Can you work these out from the drawing? Everything is in mm from the part's minimum corner. A direction names the side the tool comes from. Coordinates: 2 decimals unless noted, no trailing zeros. Loops run counter-clockwise (first coordinate to the right, second up) from the corner with the lowest first, then second, coordinate; pieces in that order, holes last. Notation, with made-up numbers: (-4.5, 70) - (42.5, 70) arc R16 cw to (42.5, 97) - close; hole circle Ø1 at (34, -26). An arc over 180 degrees is marked (long way). One line per question, with ' | ' between items. Start each with the question number.
1. I want a section at A-A, the plane x = 82. Write out the boundary of the cut face in (y, z), then the cut area to 3 significant figures.
2. I'm going to push a flat-ended pin straight in: P1, Ø5, axis at x = 55.5, y = 41.5, coming from the +Z side. Where does the tip first touch, or does it pass through?
3. Which directions (+Z, -Z, +X, -X, +Y, -Y) give clear straight access to the entire face, cutting with the end or side of a thin tool? Please do the marked faces 1 and 2.
4. We'd pull the mould along Y, two halves only. Please class the marked faces 3, 4 and 5: pulls with the +Y half, pulls with the -Y half, needs draft (parallel to the pull), parting line crosses it, or undercut.
5. I want a section at C-C, the plane z = 10.5. Write out the boundary of the cut face in (x, y).
6. Please list where these lines run through material, in increasing order: L1, parallel to Y at x = 72.5, z = 9.5; L2, parallel to X at y = 42.5, z = 1.75; L3, parallel to X at y = 49.5, z = 2.25. Write a range as [from, to].
7. I want a section at B-B, the plane y = 31. Write out the boundary of the cut face in (x, z), then the cut area to 3 significant figures.
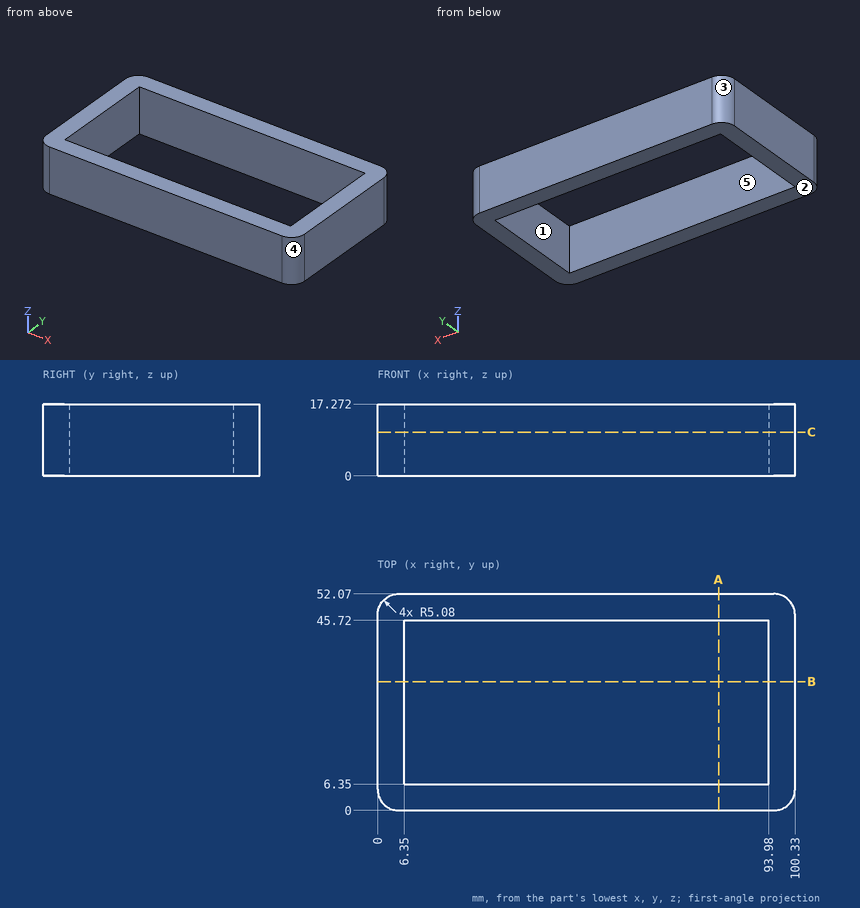
Results are:
1) outline: (0, 0) - (6.35, 0) - (6.35, 17.27) - (0, 17.27) - close; (45.72, 0) - (52.07, 0) - (52.07, 17.27) - (45.72, 17.27) - close | area: 219 mm2
2) P1: passes through
3) face 1: +Z, -Z | face 2: -Z, +X, -X, +Y, -Y
4) face 3: pulls with the +Y half | face 4: pulls with the -Y half | face 5: undercut
5) outline: (0, 5.08) arc R5.08 ccw to (5.08, 0) - (95.25, 0) arc R5.08 ccw to (100.33, 5.08) - (100.33, 46.99) arc R5.08 ccw to (95.25, 52.07) - (5.08, 52.07) arc R5.08 ccw to (0, 46.99) - close; hole (6.35, 6.35) - (93.98, 6.35) - (93.98, 45.72) - (6.35, 45.72) - close
6) L1: y = [0, 6.35], [45.72, 52.07] | L2: x = [0, 6.35], [93.98, 100.33] | L3: x = [0.66, 99.67]
7) outline: (0, 0) - (6.35, 0) - (6.35, 17.27) - (0, 17.27) - close; (93.98, 0) - (100.33, 0) - (100.33, 17.27) - (93.98, 17.27) - close | area: 219 mm2
